Source: CAD feature listing. Evaluate the final solid. Frame: model axes, mm. A direction names the side the tool comes from. Round coordinates to 2 decimals unless told otherwise and drop trailing zeros. Order: outer loops, then holes, each group sorted by start corner. A loop starts at its lowest first (then second) coordinate and runs counter-clockwise, first axis right, second up. Notation, with made-up numbers: (83.25, -5) - (126.25, -5) arc R14 cw to (126.25, 3) - close; hole circle Ø3 at (26.25, 10). An arc over 180 degrees is marked (long way). Put each result on its own line as item: value. Start each with the question number.
1) Section C-C on y = 123. Output: boundary loops of the cut face in (x, z).
2) Section A-A on z = 11.5. Output: boundary loops of the cut face in (x, y), then the cut area to 3 significant figures.
3) Mould query, pull axis Z, two halves, no side actions, for faces 1 (the face through (0, -3, 19.05)), 2 (the face through (-1.72, -217.3, 18.01)), 3 (the face through (0, -3, 16.942)), 4 (the face through (-16.942, -3, 0)). Classes: +Z half, -Z half, draft (parallel to the pull), parting line (faces both ways), or undercut.
4) Contact query for a flat-ended pin moving along its axis: P1, Ø20.5, axis at x = 0, y = -209.55, coming from the +Z side. Output: stop coordinate, or through.
5) Section D-D on y = 209.55. Output: boundary loops of the cut face in (x, z).
6) Line query: probe 1 along X at (y, z) = (155, 7.5); probe 2 along Y at (x, z) = (0, 18). Output: solid intervals per line, ascending. Write a range as [from, to].
7) Access query for faces 5 (the face through (0, -3, -19.05)), 6 (the face through (0, -3, -16.942)). Directions: +Z, -Z, +X, -X, +Y, -Y. A direction counts if a zero-diameter tool reaches every point of the face in a straight line with its end or side. Return the directions, or none.
8) Section B-B on x = 0. Output: boundary loops of the cut face in (y, z), then the cut area to 3 significant figures.
```python
from build123d import *

# Parameters (mm, degrees)
F0_W     = 38.1
F0_H     = 38.1
F0_W_2   = 33.8836
F0_H_2   = 33.8836
F1_DEPTH = 228.6
F3_DEPTH = 38.101
F4_R     = 7.9375
F5_DEPTH = 2.1082


with BuildPart() as f1:
    # F0 (on Front) → F1 (new body, symmetric)
    with BuildSketch(Plane.XZ):
        Rectangle(F0_W, F0_H)
        Rectangle(F0_W_2, F0_H_2, mode=Mode.SUBTRACT)
    extrude(amount=F1_DEPTH, both=True)

    # F2 (on face) → F3 (cut, through all)
    with BuildSketch(Plane.YZ.offset(19.05)):
        Polygon((-190.5, -19.05), (-228.6, 19.05), (-228.6, -19.05), align=None)
        Polygon((228.6, -19.05), (228.6, 19.05), (190.5, -19.05), align=None)
    extrude(amount=-F3_DEPTH, mode=Mode.SUBTRACT)

    # F4 (on face) → F5 (cut, through all)
    with BuildSketch(Plane.XY.offset(19.05)):
        with Locations((0, 209.55)):
            Circle(F4_R)
        with Locations((0, -209.55)):
            Circle(F4_R)
    extrude(amount=-F5_DEPTH, mode=Mode.SUBTRACT)


solid = f1.part
```
Answer sheet:
1. outline: (-19.05, -19.05) - (19.05, -19.05) - (19.05, 19.05) - (-19.05, 19.05) - close; hole (-16.94, -16.94) - (16.94, -16.94) - (16.94, 16.94) - (-16.94, 16.94) - close
2. outline: (-19.05, -221.05) - (-16.94, -221.05) - (-16.94, 221.05) - (-19.05, 221.05) - close; (16.94, -221.05) - (19.05, -221.05) - (19.05, 221.05) - (16.94, 221.05) - close
2. area: 1,860 mm^2
3. face 1: +Z half
3. face 2: draft
3. face 3: undercut
3. face 4: undercut
4. P1: z = 19.05
5. outline: (-19.05, 0) - (-16.94, 0) - (-16.94, 16.94) - (-7.94, 16.94) - (-7.94, 19.05) - (-19.05, 19.05) - close; (7.94, 16.94) - (16.94, 16.94) - (16.94, 0) - (19.05, 0) - (19.05, 19.05) - (7.94, 19.05) - close
6. probe 1: [-19.05, -16.94], [16.94, 19.05]
6. probe 2: [-227.55, -217.49], [-201.61, 201.61], [217.49, 227.55]
7. face 5: -Z, +X, -X, +Y, -Y
7. face 6: +Y, -Y
8. outline: (-228.6, 19.05) - (-226.49, 16.94) - (-217.49, 16.94) - (-217.49, 19.05) - close; (-201.61, 16.94) - (201.61, 16.94) - (201.61, 19.05) - (-201.61, 19.05) - close; (-192.61, -16.94) - (-190.5, -19.05) - (190.5, -19.05) - (192.61, -16.94) - close; (217.49, 16.94) - (226.49, 16.94) - (228.6, 19.05) - (217.49, 19.05) - close
8. area: 1,700 mm^2
